Input: part model. Units: mm. Frame: model coordinates. Coordinates: 2 decimals unless noted, no trailing zeros. Write each loop counter-clockwise with the first axis right and the second up, starting at its lowest first coordinate (ties: lowest second). Pieces come first, ordered by that corner, then holes. Notation, with made-up numbers: M -21.5,-5 L 10.5,-5 A25 cw 10.5,22 Z; hole C -9.5,19.5 d5. An arc over 180 degrees is marked long. Write each question's results on one line, items separated by ' | '. Start each with the question number.
1. First-contact query: pin 1 (6.5 mm diameter, centred on x = -65.5, z = 0, fed in from -Y). Flat tip, straight axial feed; report the tip coordinate or a pass-through.
2. Section query C-C, the plane y = -1.9. Output: boundary loops of the cut face in (x, z), and give its area (3 significant figures).
3. Section query A-A, the plane z = 0. Output: boundary loops of the cut face in (x, y).
4. Ray query, probe 1 along Z at (x, y) = (-65.5, -3.15); probe 2 along X at (y, z) = (-5.65, 1.5); probe 3 along X at (y, z) = (-5.3, -2.75). Return the intervals inside material, ascending.
5. Section query B-B, the plane x = 41.5. Output: boundary loops of the cut face in (y, z).
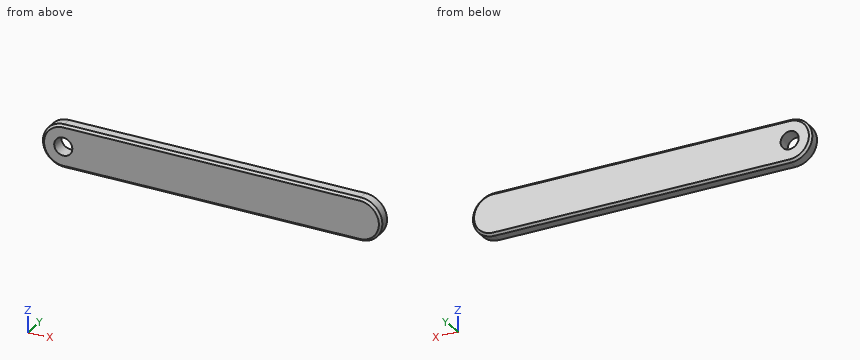
```python
from build123d import *

# Parameters (mm, degrees)
F0_R     = 4
F1_DEPTH = 6
F2_SIZE  = 1


with BuildPart() as f1:
    # F0 (on Front) → F1 (new body)
    with BuildSketch(Plane.XZ):
        with BuildLine():
            Line((65.5, 9.5), (-65.5, 9.5))
            ThreePointArc((-65.5, 9.5), (-75, 0), (-65.5, -9.5))
            Line((-65.5, -9.5), (65.5, -9.5))
            ThreePointArc((65.5, -9.5), (75, 0), (65.5, 9.5))
        make_face()
        with Locations((-65.5, 0)):
            Circle(F0_R, mode=Mode.SUBTRACT)
    extrude(amount=F1_DEPTH)

    # F2
    f2_edges = [f1.edges().sort_by_distance(p)[0] for p in [
        (0, -6, -9.5),
        (0, 0, -9.5),
    ]]
    chamfer(f2_edges, length=F2_SIZE)


solid = f1.part
```
Answer:
1) pin 1: through
2) outline: M -65.5,-9.5 L 65.5,-9.5 A9.5 ccw 65.5,9.5 L -65.5,9.5 A9.5 ccw Z; hole C -65.5,0 d8 | area: 2,720 mm^2
3) outline: M -75,-5 L -74,-6 L -69.5,-6 L -69.5,0 L -74,0 L -75,-1 Z; M -61.5,-6 L 74,-6 L 75,-5 L 75,-1 L 74,0 L -61.5,0 Z
4) probe 1: -9.5 to -4, 4 to 9.5 | probe 2: -74.22 to -69.21, -61.79 to 74.22 | probe 3: -74.28 to -68.4, -62.6 to 74.28
5) outline: M -6,-8.5 L -5,-9.5 L -1,-9.5 L 0,-8.5 L 0,8.5 L -1,9.5 L -5,9.5 L -6,8.5 Z
